Job drawing, mm, ordinate dimensions from the low corner. One solid piece. A direction names the side the tool comes from. Round coordinates to 2 decimals unless told otherwise and drop trailing zeros. Loops run counter-clockwise (first coordinate to the right, second up) from the corner with the lowest first, then second, coordinate; pieces in that order, holes last.
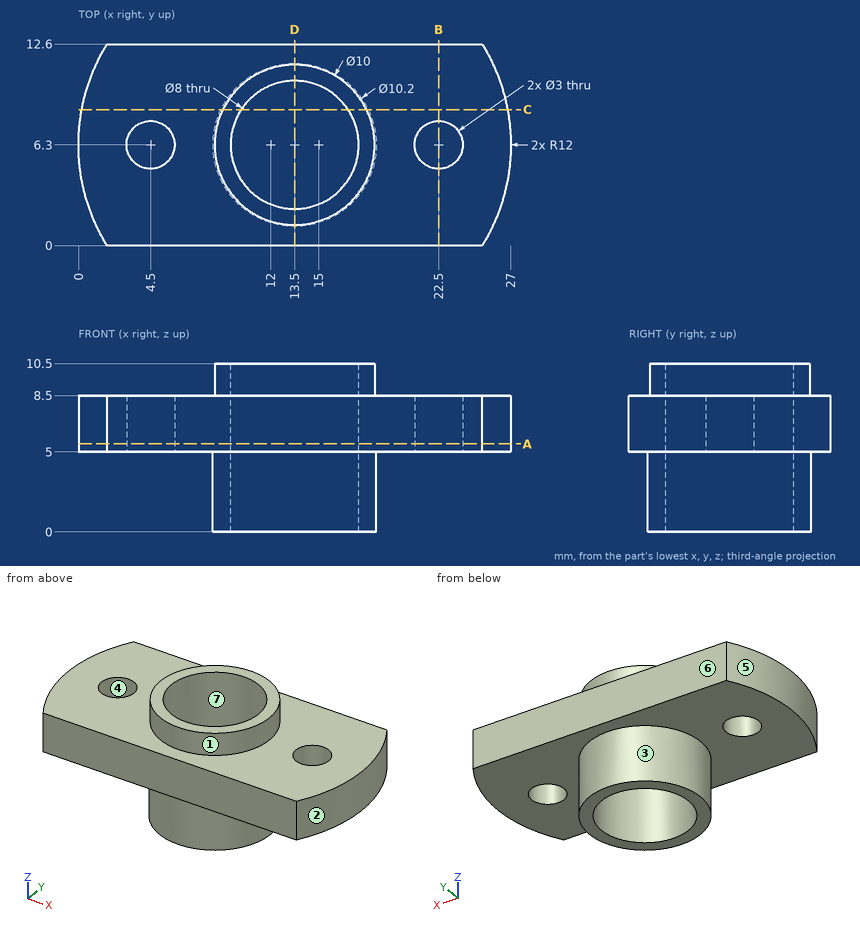
1) Wall check: line 1 along Y through (x, z) = (22.5, 6.3); line 2 along Y through (x, z) = (13.5, 7.5); line 3 along Z through (x, y) = (2, 2). Give the ranges that are in metal, low to high.
Values:
line 1: y = 0 to 4.8, 7.8 to 12.6
line 2: y = 0 to 2.3, 10.3 to 12.6
line 3: z = 5 to 8.5
2) Slice it at B-B, the plane x = 22.5. Give the cut face in (y, z).
Values:
outline: (0, 5) - (4.8, 5) - (4.8, 8.5) - (0, 8.5) - close; (7.8, 5) - (12.6, 5) - (12.6, 8.5) - (7.8, 8.5) - close
3) Tool access for the marked faces 1, 2 and 3: list every direction of +Z, -Z, +X, -X, +Y, -Y with a clear straight run to the whole face (end or side of a thin tool).
Values:
face 1: +Z
face 2: +Z, -Z, +X
face 3: -Z
4) Drop flat-ended pins along their axis: pin 1 Ø1 at (y, z) = (11, 2) entering from +X; pin 2 Ø6.5 at (x, y) = (13.5, 6.3) entering from -Z; pin 3 Ø5 at (x, y) = (4.5, 6.3) entering from -Z; pin 4 Ø4 at (y, z) = (2.5, 5.5) entering from +X. Give the stop position or say it passes through.
Values:
pin 1: stops at x = 16.39
pin 2: passes through
pin 3: stops at z = 5
pin 4: stops at x = 26.86
5) Slice it at C-C, the plane y = 8.5. Give the cut face in (x, z).
Values:
outline: (0.2, 5) - (8.9, 5) - (8.9, 0) - (10.16, 0) - (10.16, 10.5) - (9.01, 10.5) - (9.01, 8.5) - (0.2, 8.5) - close; (16.84, 0) - (18.1, 0) - (18.1, 5) - (26.8, 5) - (26.8, 8.5) - (17.99, 8.5) - (17.99, 10.5) - (16.84, 10.5) - close
6) Mould opens along Y. For the marked faces 4, 5, 6 and 7 say: released by +Y, released by -Y, zero draft, split by the parting line, or undercut.
Values:
face 4: undercut
face 5: split by the parting line
face 6: released by +Y
face 7: undercut
7) Slice it at A-A, the plane z = 5.5. Give the cut face in (x, y).
Values:
outline: (1.79, 0) - (25.21, 0) arc R12 ccw to (25.21, 12.6) - (1.79, 12.6) arc R12 ccw to start; hole circle Ø3 at (4.5, 6.3); hole circle Ø8 at (13.5, 6.3); hole circle Ø3 at (22.5, 6.3)
8) Slice it at D-D, the plane x = 13.5. Give the cut face in (y, z), then the cut area to 3 significant figures.
Values:
outline: (0, 5) - (1.2, 5) - (1.2, 0) - (2.3, 0) - (2.3, 10.5) - (1.3, 10.5) - (1.3, 8.5) - (0, 8.5) - close; (10.3, 0) - (11.4, 0) - (11.4, 5) - (12.6, 5) - (12.6, 8.5) - (11.3, 8.5) - (11.3, 10.5) - (10.3, 10.5) - close
area: 31.1 mm2
